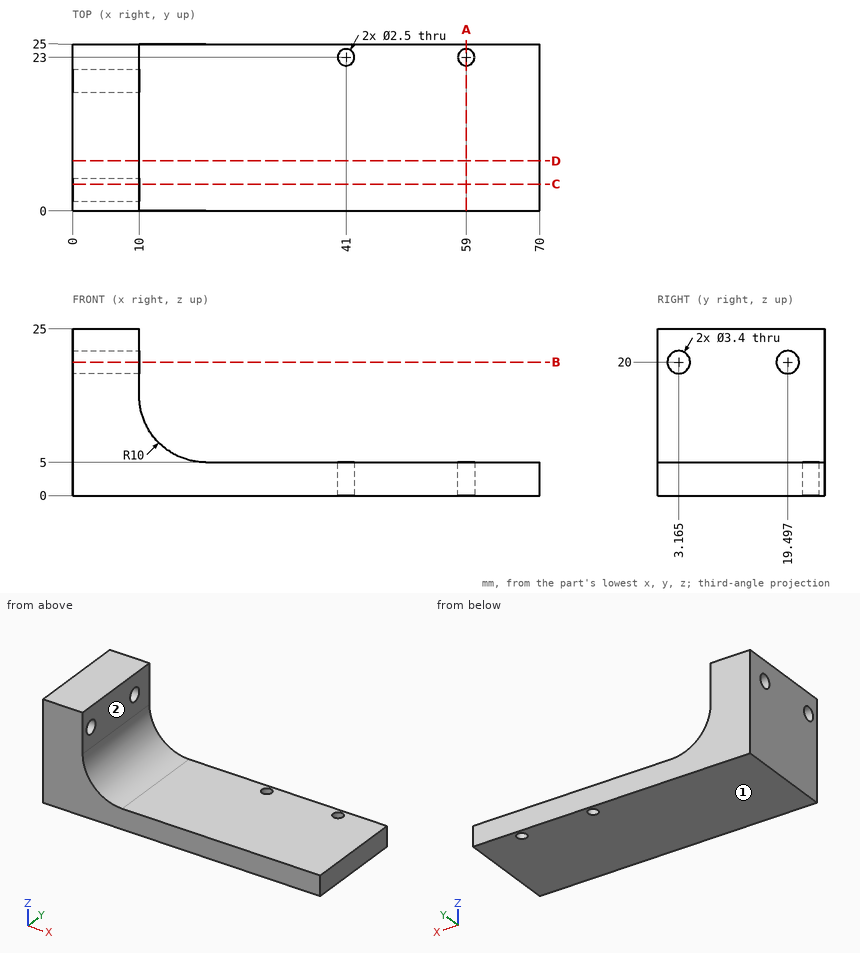
Geometry: see drawing. Coordinates: mm, zero at the bounding-box minimum. A direction names the side the tool comes from. Round coordinates to 2 decimals unless told otherwise and drop trailing zeros. Order: outer loops, then holes, each group sorted by start corner. A loop starts at its lowest first (then second) coordinate and runs counter-clockwise, first axis right, second up. Notation, with made-up numbers: (44.25, -14.75) - (60.25, -14.75) arc R6 ccw to (60.25, -9.75) - close; hole circle Ø1 at (60, 70.25). An arc over 180 degrees is marked (long way). One line per question, with ' | ' between items. Start each with the question number.
1) Ray query, probe 1 along Y at (x, z) = (5.75, 20) (3 decimals); probe 2 along Y at (x, z) = (41, 3.15); probe 3 along Z at (x, y) = (28, 12). Return the intervals inside material, ascending.
2) Cut plane B-B, the plane z = 20. Return the cut outline in (x, y) (3 decimals).
3) Cut plane C-C, the plane y = 4. Return the cut outline in (x, z), then the cut area to 3 significant figures.
4) Cut plane D-D, the plane y = 7.5. Return the cut outline in (x, z).
5) Cut plane A-A, the plane x = 59. Return the cut outline in (y, z), then the cut area to 4 significant figures.
6) Contact query for flat-ended pins moving along their axis: P1, Ø3, axis at x = 41, y = 23, coming from the +Z side; P2, Ø2, axis at x = 15, y = 3.5, coming from the +Z side; P3, Ø3, axis at y = 21.5, z = 19, coming from the -X side; P4, Ø11, axis at y = 16.5, z = 22.5, coming from the +X side. Output: stop coordinate, or through.
7) Set-up query: the marked faces 1 and 2. Return all of +Z, -Z, +X, -X, +Y, -Y with unobstructed straight access to the full face (end or side cutting, diameter ignored); none if empty.
Worked out:
1) probe 1: y = 0 to 1.465, 4.865 to 17.797, 21.197 to 25 | probe 2: y = 0 to 21.75, 24.25 to 25 | probe 3: z = 0 to 5
2) outline: (0, 0) - (10, 0) - (10, 1.465) - (0, 1.465) - close; (0, 4.865) - (10, 4.865) - (10, 17.797) - (0, 17.797) - close; (0, 21.197) - (10, 21.197) - (10, 25) - (0, 25) - close
3) outline: (0, 0) - (70, 0) - (70, 5) - (20, 5) arc R10 cw to (10, 15) - (10, 18.52) - (0, 18.52) - close; (0, 21.48) - (10, 21.48) - (10, 25) - (0, 25) - close | area: 542 mm^2
4) outline: (0, 0) - (70, 0) - (70, 5) - (20, 5) arc R10 cw to (10, 15) - (10, 25) - (0, 25) - close
5) outline: (0, 0) - (21.75, 0) - (21.75, 5) - (0, 5) - close; (24.25, 0) - (25, 0) - (25, 5) - (24.25, 5) - close | area: 112.5 mm^2
6) P1: stops at z = 5 | P2: stops at z = 7 | P3: stops at x = 0 | P4: stops at x = 10
7) face 1: -Z, +X, -X, +Y, -Y | face 2: +Z, +X, +Y, -Y
